from build123d import *

# Parameters (mm, degrees)
SKETCH1_W               = 431.8
SKETCH1_H               = 171.45
BOSS_EXTRUDE1_DEPTH     = 85.725
CUT_EXTRUDE1_DEPTH      = 73.025
FILLET3_R               = 44.45
F_0_25_OFF_TOP_DEPTH    = 6.35
SKETCH4_W               = 431.8
SKETCH4_H               = 79.375
CUT_EXTRUDE_0_125_DEPTH = 4.445
SKETCH5_W               = 167.005
SKETCH5_H               = 66.675
F_1_8_IN_DEPTH          = 4.445
SKETCH6_W               = 427.355
SKETCH6_H               = 79.375
CUT_EXTRUDE5_DEPTH      = 4.445
SKETCH7_W               = 162.0012
SKETCH7_H               = 66.675
CUT_EXTRUDE6_DEPTH      = 4.445
FILLET5_R               = 6.35


with BuildPart() as part:
    # Sketch1 → Boss-Extrude1 (new body)
    with BuildSketch(Plane(origin=(0, 0, 0), x_dir=(1, 0, 0), z_dir=(0, 1, 0))):
        Rectangle(SKETCH1_W, SKETCH1_H)
    extrude(amount=BOSS_EXTRUDE1_DEPTH)

    # Sketch2 → Cut-Extrude1 (cut)
    with BuildSketch(Plane.XZ):
        with BuildLine():
            Line((162.16885638, 76.686434381), (-162.16885638, 76.686434381))
            ThreePointArc((-162.16885638, 76.686434381), (-193.771281353, 63.596281353), (-206.861434381, 31.99385638))
            Line((-206.861434381, 31.99385638), (-206.861434381, -31.99385638))
            ThreePointArc((-206.861434381, -31.99385638), (-193.771281353, -63.596281353), (-162.16885638, -76.686434381))
            Line((-162.16885638, -76.686434381), (162.16885638, -76.686434381))
            ThreePointArc((162.16885638, -76.686434381), (193.771281353, -63.596281353), (206.861434381, -31.99385638))
            Line((206.861434381, -31.99385638), (206.861434381, 31.99385638))
            ThreePointArc((206.861434381, 31.99385638), (193.771281353, 63.596281353), (162.16885638, 76.686434381))
        make_face()
    extrude(amount=-CUT_EXTRUDE1_DEPTH, mode=Mode.SUBTRACT)

    # Fillet3
    fillet3_edges = [part.edges().sort_by_distance(p)[0] for p in [
        (215.9, 42.8625, 85.725),
        (-215.9, 42.8625, 85.725),
        (-215.9, 42.8625, -85.725),
        (215.9, 42.8625, -85.725),
    ]]
    fillet(fillet3_edges, radius=FILLET3_R)

    # Sketch3 → 0.25 off top (cut)
    with BuildSketch(Plane(origin=(0, 85.725, 0), x_dir=(1, 0, 0), z_dir=(0, 1, 0))):
        with BuildLine():
            Line((215.9, -41.275), (215.9, 41.275))
            ThreePointArc((215.9, 41.275), (202.880896424, 72.705896424), (171.45, 85.725))
            Line((171.45, 85.725), (-171.45, 85.725))
            ThreePointArc((-171.45, 85.725), (-202.880896424, 72.705896424), (-215.9, 41.275))
            Line((-215.9, 41.275), (-215.9, -41.275))
            ThreePointArc((-215.9, -41.275), (-202.880896424, -72.705896424), (-171.45, -85.725))
            Line((-171.45, -85.725), (171.45, -85.725))
            ThreePointArc((171.45, -85.725), (202.880896424, -72.705896424), (215.9, -41.275))
        make_face()
    extrude(amount=-F_0_25_OFF_TOP_DEPTH, mode=Mode.SUBTRACT)

    # Sketch4 → 0.125 (cut)
    with BuildSketch(Plane.XY.offset(85.725)):
        with Locations((0, 39.6875)):
            Rectangle(SKETCH4_W, SKETCH4_H)
    extrude(amount=-CUT_EXTRUDE_0_125_DEPTH, mode=Mode.SUBTRACT)

    # Sketch5 → 1/8 in (cut)
    with BuildSketch(Plane.ZY.offset(215.9)):
        with Locations((-2.2225, 33.3375)):
            Rectangle(SKETCH5_W, SKETCH5_H)
    extrude(amount=-F_1_8_IN_DEPTH, mode=Mode.SUBTRACT)

    # Sketch6 → Cut-Extrude5 (cut)
    with BuildSketch(Plane(origin=(0, 0, -85.725), x_dir=(-1, 0, 0), z_dir=(0, 0, -1))):
        with Locations((-2.2225, 39.6875)):
            Rectangle(SKETCH6_W, SKETCH6_H)
    extrude(amount=-CUT_EXTRUDE5_DEPTH, mode=Mode.SUBTRACT)

    # Sketch7 → Cut-Extrude6 (cut)
    with BuildSketch(Plane(origin=(215.9, 0, 0), x_dir=(0, 0, -1), z_dir=(1, 0, 0))):
        with Locations((0.2794, 33.3375)):
            Rectangle(SKETCH7_W, SKETCH7_H)
    extrude(amount=-CUT_EXTRUDE6_DEPTH, mode=Mode.SUBTRACT)

    # Fillet5
    fillet5_edges = [part.edges().sort_by_distance(p)[0] for p in [
        (0, 79.375, -81.28),
        (0, 79.375, 81.28),
    ]]
    fillet(fillet5_edges, radius=FILLET5_R)


solid = part.part
For this review, take the finished solid that the model builds, in its own axes (mm). A direction names the side the tool comes from. Round coordinates to 2 decimals unless told otherwise and drop trailing zeros. Write each loop counter-clockwise with the first axis right and the second up, starting at its lowest first coordinate (ties: lowest second). Pieces come first, ordered by that corner, then holes. Notation, with made-up numbers: (55, 70) -> (79, 70) arc R29 ccw to (79, 107) -> close; hole circle Ø7 at (-5.5, 86). An arc over 180 degrees is marked (long way). Put each result on its own line as item: value.
Q1. To check wall thickness, follow L1, parallel to Z at x = 5, y = 62; L2, parallel to X at y = 55.5, z = -10 (3 decimals); L3, parallel to Y at x = 16, z = 53 (3 decimals). State the ranges of each line that lie inside material, in increasing order. Write a range as [from, to].
Determined:
L1: z = [-81.28, -76.69], [76.69, 81.28]
L2: x = [-211.455, -206.861], [206.861, 211.455]
L3: y = [73.025, 79.375]
Q2. Consider section C-C on z = 50. State the section outline as (x, y) points (3 decimals).
Determined:
outline: (-215.035, 66.675) -> (-211.455, 66.675) -> (-211.455, 0) -> (-203.074, 0) -> (-203.074, 73.025) -> (203.074, 73.025) -> (203.074, 0) -> (211.455, 0) -> (211.455, 66.675) -> (215.035, 66.675) -> (215.035, 79.375) -> (-215.035, 79.375) -> close
Q3. Clearance check with flat-ended pins moving along their axes: pin 1 Ø4 at (y, z) = (35, -26.5) entering from +X (3 decimals); pin 2 Ø3.5 at (x, z) = (-214.5, -23) entering from -Y (3 decimals); pin 3 Ø12 at (x, z) = (26, -25) entering from -Y (3 decimals). State where each tip first meets the part, or that it passes through.
Determined:
pin 1: stops at x = 211.455
pin 2: stops at y = 66.675
pin 3: stops at y = 73.025
Q4. The part is to be moulded in two halves that separate along X. For faces 1 (the flat face through (-2, 36, -76.686)), 2 (the flat face through (-211.455, 34, -1)), 3 (the cylindrical face through (205.671, 49.063, -69.642)), say which applies: released by +X, released by -X, zero draft, split by the parting line, or undercut.
Determined:
face 1: undercut
face 2: released by -X
face 3: released by +X
Q5. Consider section B-B on x = -105. State the section outline as (y, z) points (3 decimals), and give its area (3 significant figures).
Determined:
outline: (0, -81.28) -> (73.025, -81.28) arc R6.35 ccw to (79.375, -74.93) -> (79.375, 74.93) arc R6.35 ccw to (73.025, 81.28) -> (0, 81.28) -> (0, 76.686) -> (73.025, 76.686) -> (73.025, -76.686) -> (0, -76.686) -> close
area: 1,690 mm^2
Q6. Consider section D-D on x = 173.5. State the section outline as (y, z) points (3 decimals), and give its area (3 significant figures).
Determined:
outline: (0, -81.28) -> (73.025, -81.28) arc R6.35 ccw to (79.375, -74.93) -> (79.375, 74.93) arc R6.35 ccw to (73.025, 81.28) -> (0, 81.28) -> (0, 75.226) -> (73.025, 75.226) -> (73.025, -75.226) -> (0, -75.226) -> close
area: 1,900 mm^2
Q7. Machinability: for faces 4 (the flat face through (215.9, 73, 1)), 5 (the cylindrical face through (-194.117, 36.001, -63.247)), 6 (the flat face through (211.455, 34, 1)), which of the approach directions +Z, -Z, +X, -X, +Y, -Y give a long, thin tool a straight path to every point of the face, cutting with its end or side? Answer none if there is none.
Determined:
face 4: +Z, -Z, +X, +Y, -Y
face 5: -Y
face 6: +Z, -Z, +X, -Y
Q8. Consider section A-A on y = 34. State the section outline as (x, z) points (3 decimals).
Determined:
outline: (-211.455, -60.65) arc R44.45 ccw to (-190.825, -81.28) -> (190.825, -81.28) arc R44.45 ccw to (211.455, -60.65) -> (211.455, 60.65) arc R44.45 ccw to (190.825, 81.28) -> (-190.825, 81.28) arc R44.45 ccw to (-211.455, 60.65) -> close; hole (-206.861, -31.994) arc R44.693 ccw to (-162.169, -76.686) -> (162.169, -76.686) arc R44.693 ccw to (206.861, -31.994) -> (206.861, 31.994) arc R44.693 ccw to (162.169, 76.686) -> (-162.169, 76.686) arc R44.693 ccw to (-206.861, 31.994) -> close
